Part model, mm, in its own coordinate system. A direction names the side the tool comes from. Round coordinates to 2 decimals unless told otherwise and drop trailing zeros. Write each loop counter-clockwise with the first axis right and the second up, starting at its lowest first coordinate (ties: lowest second). Pieces come first, ordered by that corner, then holes. Notation, with made-up numbers: M 62,53 L 112,53 A21 ccw 112,86 Z; hole C -32.75,-15.75 d7. An arc over 180 degrees is marked long. Answer as a JSON object with one key per item and string values. Group by question number.
1. Two-plate mould, pull along X, no slides. Class faces 5 (the face through (-14, 0, -23)), 6 (the face through (4.762, 3, -22)), 7 (the face through (-18.361, 15.653, -27.264)): +X half, -X half, draft (parallel to the pull), parting line (faces both ways), or undercut.
2. Band-saw the part on D-D, the plane z = -7.5. Write the cut outline in (x, y), plus the area to 3 significant figures.
3. Drop flat-ended pins along their axis: pin 1 (8 mm diameter, centred on x = -34, y = 22, fed in from +Z); pin 2 (2 mm diameter, centred on y = 14, z = -4, fed in from +X); pin 3 (8 mm diameter, centred on x = -15.5, y = 25.5, fed in from -Z). Give the stop position or say it passes through.
4. Band-saw the part on C-C, the plane x = -39. Write the cut outline in (y, z), plus the area to 3 significant figures.
5. Drill centre lines: line 1 (Z direction, x = -31.5, y = 18); line 2 (Y direction, x = -1.5, z = -38); line 3 (Z direction, x = -17, y = 19.5). Where is each one in solid material? Low to high. Write a range as from..to.
6. Which spindle directions (+Z, -Z, +X, -X, +Y, -Y) get a long thin tool onto all of the face, cutting with end or side? Do faces 1 (the face through (-1.588, 19, -22)), 2 (the face through (-23, 19, -1.588)), 3 (the face through (-46.776, 18.701, -30.155)), 4 (the face through (-22, 19, -42.862)). Say none if no direction does.
7. Band-saw the part on A-A, the plane x = -27. Write the cut outline in (y, z).
Autodesk Inventor part; units mm, degrees
ref_plane "YZ Plane" through (0, 0, 0) normal (1, 0, 0) x (0, 1, 0)
ref_plane "XZ Plane" through (0, 0, 0) normal (0, 1, 0) x (-1, 0, 0)
ref_plane "XY Plane" through (0, 0, 0) normal (0, 0, 1) x (1, 0, 0)
sketch "Sketch1" plane through (0, 0, 0) normal (0, 1, 0) x (-1, 0, 0)
  line L0 (0, 0) -> (42.8625, 0)
  line L1 (42.8625, 0) -> (42.8625, -44.45)
  line L2 (42.8625, -44.45) -> (0, -44.45)
  line L3 (0, -44.45) -> (0, 0)
  dimension "d0" = 44.45
  dimension "d1" = 42.8625
extrude "Extrusion1" add sketch "Sketch1" along normal blind 31.75
sketch "Sketch2" plane through (-42.8625, 0, 0) normal (0, 0, 1) x (1, 0, 0)
  line L0 (0, 0) -> (0, 31.75)
  line L1 (42.8625, 0) -> (42.8625, 31.75)
  line L2 (42.8625, 0) -> (0, 0)
  line L3 (0, 6.35) -> (42.8625, 6.35)
  line L4 (42.8625, 6.35) -> (42.8625, 31.75)
  line L5 (42.8625, 31.75) -> (0, 31.75)
  line L6 (0, 31.75) -> (0, 6.35)
  dimension "d5" = 6.35
extrude "Extrusion2" cut sketch "Sketch2" against normal blind 1.5875 contours L0 L5 L1 L3
sketch "Sketch3" plane through (0, 0, 0) normal (1, 0, 0) x (0, 0, -1)
  line L0 (1.5875, 31.75) -> (1.5875, 6.35)
  line L1 (44.45, 0) -> (44.45, 31.75)
  line L2 (1.5875, 6.35) -> (44.45, 6.35)
  line L3 (44.45, 6.35) -> (44.45, 31.75)
  line L4 (44.45, 31.75) -> (1.5875, 31.75)
  line L5 (1.5875, 31.75) -> (1.5875, 6.35)
  point P0 (0, 0)
extrude "Extrusion3" cut sketch "Sketch3" against normal blind 1.5875
sketch "Sketch9" plane through (0, 31.75, 0) normal (0, 1, 0) x (1, 0, 0)
  line L0 (0, 44.45) -> (0, 0)
  line L1 (-1.5875, 44.45) -> (0, 44.45)
  point P0 (-22.225, 22.225)
  point P1 (-42.8625, 44.45)
  dimension "d23" = 22.225
  dimension "d24" = 22.225
hole "Hole1" at (-22.225, 31.75, -22.225) direction (0, -1, 0) diameter 12.7 end through all
sketch "Sketch19" plane through (0, 0, -44.45) normal (0, 0, -1) x (-1, 0, 0)
  line L0 (1.5875, 31.75) -> (42.8625, 31.75)
  line L1 (1.5875, 6.35) -> (42.8625, 6.35)
  line L2 (1.5875, 31.75) -> (42.8625, 31.75)
  line L3 (42.8625, 31.75) -> (42.8625, 6.35)
  line L4 (42.8625, 6.35) -> (1.5875, 6.35)
  line L5 (1.5875, 6.35) -> (1.5875, 31.75)
  point P0 (0, 0)
extrude "Extrusion14" cut sketch "Sketch19" against normal blind 1.5875
sketch "Sketch20" plane through (-42.8625, 0, -44.45) normal (-1, 0, 0) x (0, 0, 1)
  circle A0 centre (22.225, 19.05) radius 7.9375
  line L0 (44.45, 0) -> (0, 0)
  line L1 (44.45, 0) -> (44.45, 6.35)
  dimension "d59" = 15.875
  dimension "d60" = 19.05
  dimension "d61" = 22.225
extrude "Extrusion15" add sketch "Sketch20" along normal blind 7.9375
sketch "Sketch21" plane through (0, 0, -44.45) normal (0, 0, -1) x (-1, 0, 0)
  line L0 (42.8625, 6.35) -> (0, 6.35)
  line L1 (0, 0) -> (0, 6.35)
  line L2 (42.8625, 0) -> (0, 0)
  line L3 (42.8625, 0) -> (42.8625, 6.35)
  point P0 (0, 0)
extrude "Extrusion16" add sketch "Sketch21" along normal blind 4.7625
sketch "Sketch22" plane through (-42.8625, 0, 0) normal (0, 0, 1) x (1, 0, 0)
  line L0 (42.8625, 6.35) -> (0, 6.35)
  line L1 (0, 0) -> (0, 6.35)
  line L2 (42.8625, 0) -> (0, 0)
  line L3 (42.8625, 0) -> (42.8625, 6.35)
extrude "Extrusion17" add sketch "Sketch22" along normal blind 4.7625
sketch "Sketch23" plane through (0, 0, -49.2125) normal (1, 0, 0) x (0, 0, -1)
  line L0 (0, 6.35) -> (-53.975, 6.35)
  line L1 (-53.975, 0) -> (-53.975, 6.35)
  line L2 (0, 0) -> (-53.975, 0)
  line L3 (0, 6.35) -> (0, 0)
  point P0 (-49.2125, 0)
extrude "Extrusion18" add sketch "Sketch23" along normal blind 4.7625
properties part number "WackyPlug1.75"
Worked answers:
{
 "1": {"face 5": "draft", "face 6": "+X half", "face 7": "undercut"},
 "2": {"outline": "M -42.86,0 L 4.76,0 L 4.76,6.35 L -1.59,6.35 L -1.59,31.75 L -42.86,31.75 Z", "area": "1,350 mm^2"},
 "3": {"pin 1": "stops at z = -1.59", "pin 2": "stops at x = -1.59", "pin 3": "stops at z = -42.86"},
 "4": {"outline": "M 0,-49.21 L 6.35,-49.21 L 6.35,-42.86 L 31.75,-42.86 L 31.75,-1.59 L 6.35,-1.59 L 6.35,4.76 L 0,4.76 Z", "area": "1,390 mm^2"},
 "5": {"line 1": "z = -42.86..-1.59", "line 2": "y = 0..6.35", "line 3": "z = -42.86..-25.83, -18.62..-1.59"},
 "6": {"face 1": "+Z, -Z, +X, +Y", "face 2": "+Z, +X, -X, +Y", "face 3": "-X", "face 4": "-Z, +X, -X, +Y"},
 "7": {"outline": "M 0,-49.21 L 6.35,-49.21 L 6.35,-42.86 L 31.75,-42.86 L 31.75,-26.41 L 0,-26.41 Z; M 0,-18.04 L 31.75,-18.04 L 31.75,-1.59 L 6.35,-1.59 L 6.35,4.76 L 0,4.76 Z"}
}
